Read the model definition and answer for the solid it produces. Units are mm, in the model's axes. A direction names the side the tool comes from. Round coordinates to 2 decimals unless told otherwise and drop trailing zeros. Write each loop counter-clockwise with the first axis right and the second up, starting at its lowest first coordinate (ties: lowest second). Pieces come first, ordered by that corner, then holes. Notation, with made-up numbers: (-39, 43.5) - (6, 43.5) arc R19 ccw to (6, 68.5) - close; hole circle Ø6 at (-25.75, 71). An arc over 180 degrees is marked (long way). Answer as CSV lines item,"result". Start each with the question number.
1) For a pull along X with two mould halves and no side action, classify faces 1 (the flat face through (0, -34, 0)), 2 (the flat face through (40.782, -47, 4)), 3 (the flat face through (-39.218, -45, 4)), 4 (the flat face through (-19.218, 9, 4)) as +X half, -X half, draft (parallel to the pull), parting line (faces both ways), or undercut.
2) Each of these flat-tipped pins is pushed along its axis until it touches: pin 1 (4 mm diameter, centred on y = 10, z = 2, fed in from +X); pin 2 (2.5 mm diameter, centred on y = 11, z = 2.5, fed in from -X); pin 3 (2.5 mm diameter, centred on x = -37.5, z = 6, fed in from +Y). Where does it stop, or does it pass through?
3) Which of the six approach directions +Z, -Z, +X, -X, +Y, -Y give full straight-line access (tool end or side, diameter ignored) to faces 5 (the flat face through (-27, 21.968, 4)), 6 (the flat face through (38, -1.032, 4)), 7 (the flat face through (-37, -1.032, 4)), 8 (the flat face through (1, -1.032, 4))?
4) Find section C-C on y = -83. Determine the outline of the cut face in (x, z), then the cut area to 3 significant figures.
5) Find section B-B on z = 2.5. Determine the outline of the cut face in (x, y).
6) Find section A-A on y = 13.5. Determine the outline of the cut face in (x, z).
7) Consider line 1 along Y through (x, z) = (18, 3.5); line 2 along X through (y, z) = (7.5, 6); line 3 along X through (y, z) = (-85.5, 0.5). Determine where each line is inside the solid, lowest interval first.
8) Find section D-D on x = 1. Determine the outline of the cut face in (y, z).
from build123d import *

# Parameters (mm, degrees)
F1_DEPTH = 8


with BuildPart() as f1:
    # F0 (on Top) → F1 (new body)
    with BuildSketch(Plane.XY):
        with BuildLine():
            Line((-34.218354, -1.032101), (-39.218354, -1.032101))
            Line((-39.218354, -1.032101), (-39.218354, -91.032101))
            Line((-39.218354, -91.032101), (-14.218354, -91.032101))
            ThreePointArc((-14.218354, -91.032101), (0.781646, -76.032101), (15.781646, -91.032101))
            Line((15.781646, -91.032101), (40.781646, -91.032101))
            Line((40.781646, -91.032101), (40.781646, -1.032101))
            Line((40.781646, -1.032101), (35.781646, -1.032101))
            Line((35.781646, -1.032101), (35.781646, 18.967899))
            ThreePointArc((35.781646, 18.967899), (34.902966, 21.089219), (32.781646, 21.967899))
            Line((32.781646, 21.967899), (23.781646, 21.967899))
            ThreePointArc((23.781646, 21.967899), (21.660325, 21.089219), (20.781646, 18.967899))
            Line((20.781646, 18.967899), (20.781646, -1.032101))
            Line((20.781646, -1.032101), (-17.203856, -1.032101))
            Line((-17.203856, -1.032101), (-19.218354, -1.032101))
            Line((-19.218354, -1.032101), (-19.218354, 18.967899))
            ThreePointArc((-19.218354, 18.967899), (-20.097034, 21.089219), (-22.218354, 21.967899))
            Line((-22.218354, 21.967899), (-31.218354, 21.967899))
            ThreePointArc((-31.218354, 21.967899), (-33.339675, 21.089219), (-34.218354, 18.967899))
            Line((-34.218354, 18.967899), (-34.218354, -1.032101))
        make_face()
    extrude(amount=F1_DEPTH)


solid = f1.part
Check values:
1,face 1,"draft"
1,face 2,"+X half"
1,face 3,"-X half"
1,face 4,"undercut"
2,pin 1,"stops at x = 35.78"
2,pin 2,"stops at x = -34.22"
2,pin 3,"stops at y = -1.03"
3,face 5,"+Z, -Z, +X, -X, +Y"
3,face 6,"+Z, -Z, +X, +Y"
3,face 7,"+Z, -Z, -X, +Y"
3,face 8,"+Z, -Z, +Y"
4,outline,"(-39.22, 0) - (-11.89, 0) - (-11.89, 8) - (-39.22, 8) - close; (13.45, 0) - (40.78, 0) - (40.78, 8) - (13.45, 8) - close"
4,area,"437 mm^2"
5,outline,"(-39.22, -91.03) - (-14.22, -91.03) arc R15 cw to (15.78, -91.03) - (40.78, -91.03) - (40.78, -1.03) - (35.78, -1.03) - (35.78, 18.97) arc R3 ccw to (32.78, 21.97) - (23.78, 21.97) arc R3 ccw to (20.78, 18.97) - (20.78, -1.03) - (-19.22, -1.03) - (-19.22, 18.97) arc R3 ccw to (-22.22, 21.97) - (-31.22, 21.97) arc R3 ccw to (-34.22, 18.97) - (-34.22, -1.03) - (-39.22, -1.03) - close"
6,outline,"(-34.22, 0) - (-19.22, 0) - (-19.22, 8) - (-34.22, 8) - close; (20.78, 0) - (35.78, 0) - (35.78, 8) - (20.78, 8) - close"
7,line 1,"y = -91.03 to -1.03"
7,line 2,"x = -34.22 to -19.22, 20.78 to 35.78"
7,line 3,"x = -39.22 to -13.16, 14.72 to 40.78"
8,outline,"(-76.03, 0) - (-1.03, 0) - (-1.03, 8) - (-76.03, 8) - close"
